Build history of the part. All positions in model axes, mm. Give positions to 0.01 mm unless a question says otherwise; leave off trailing zeros. Order: outer loops, then holes, each group sorted by start corner. A loop starts at its lowest first (then second) coordinate and runs counter-clockwise, first axis right, second up. Notation, with made-up numbers: M 37.25,-32 L 62.25,-32 A28 ccw 62.25,-5 Z; hole C 12.25,77.5 d9. An arc over 180 degrees is marked long. Answer as CSV lines item,"result".
from build123d import *

# Parameters (mm, degrees)
SKETCH1_R      = 1.1303
SKETCH1_R_2    = 1.130299999
EXTRUDE1_DEPTH = 12.7
SKETCH2_R      = 3.810000001
SKETCH2_R_2    = 1.130299999
EXTRUDE2_DEPTH = 17.145


with BuildPart() as part:
    # Sketch1 → Extrude1 (new body)
    with BuildSketch(Plane.XY):
        with BuildLine():
            Line((286.542223003, 20.061166103), (324.474632327, -15.639737839))
            ThreePointArc((324.474632327, -15.639737839), (329.813577235, -15.525304753), (329.793827414, -10.185170147))
            Line((329.793827414, -10.185170147), (297.063524693, 22.885170148))
            ThreePointArc((297.063524693, 22.885170148), (291.649695142, 22.043861139), (286.542223003, 20.061166103))
        make_face()
        with Locations((296.613066371, 17.154306926)):
            Circle(SKETCH1_R, mode=Mode.SUBTRACT)
        with Locations((327.08586457, -12.865289034)):
            Circle(SKETCH1_R_2, mode=Mode.SUBTRACT)
    extrude(amount=EXTRUDE1_DEPTH)

    # Sketch2 → Extrude2 (add)
    with BuildSketch(Plane.XY):
        with Locations(Location((327.08586457, -12.865289034, 0), (0, 0, 226.735854521))):
            Circle(SKETCH2_R)
        with Locations((327.08586457, -12.865289034)):
            Circle(SKETCH2_R_2, mode=Mode.SUBTRACT)
    extrude(amount=EXTRUDE2_DEPTH)


solid = part.part
Item 1: Probe line 1 along Z through (x, y) = (301, 9); line 2 along X through (y, z) = (-13.5, 7.5); line 3 along X through (y, z) = (-5, 1). List the from-to ranges inside material, lowest first. Write a range as from..to.
Geometry says:
line 1,"z = 0..12.7"
line 2,"x = 322.2..326.15, 328.02..330.84"
line 3,"x = 313.17..324.66"
Item 2: Band-saw the part on D-D (x = 307). Give the cut face in (y, z).
Geometry says:
outline,"M 0.81,0 L 12.85,0 L 12.85,12.7 L 0.81,12.7 Z"
Item 3: Pull direction Y, two halves, no side cores. Call faces 1 (the cylindrical face through (330.18, -15.09, 10.36)), 2 (the flat face through (310, 5, 0)), 3 (the cylindrical face through (328.13, -13.3, 8.45)): released by +Y, released by -Y, zero draft, split by the parting line, or undercut.
Geometry says:
face 1,"split by the parting line"
face 2,"zero draft"
face 3,"undercut"
Item 4: Band-saw the part on A-A (z = 2.5). Give the cut face in (x, y).
Geometry says:
outline,"M 286.54,20.06 L 324.47,-15.64 A3.81 ccw 329.79,-10.19 L 297.06,22.89 A25.4 ccw Z; hole C 296.61,17.15 d2.26; hole C 327.09,-12.87 d2.26"
Item 5: Band-saw the part on C-C (z = 14.25). Give the cut face in (x, y), and give its area (3 significant figures).
Geometry says:
outline,"C 327.09,-12.87 d7.62; hole C 327.09,-12.87 d2.26"
area,"41.6 mm2"
Item 6: Drop flat-ended pins along their axis: pin 1 (4 mm diameter, centred on x = 319, z = 2.5, fed in from +Y); pin 2 (2 mm diameter, centred on x = 312, z = 2, fed in from -Y); pin 3 (4 mm diameter, centred on x = 313, z = 11.5, fed in from +Y). Give the stop position or say it passes through.
Geometry says:
pin 1,"stops at y = 2.74"
pin 2,"stops at y = -4.84"
pin 3,"stops at y = 8.8"
Item 7: Band-saw the part on B-B (y = -13.5). Give the cut face in (x, z) (3 decimals), and give its area (3 significant figures).
Geometry says:
outline,"M 322.201,0 L 326.151,0 L 326.151,17.145 L 323.329,17.145 L 323.329,12.7 L 322.201,12.7 Z; M 328.021,0 L 330.843,0 L 330.843,17.145 L 328.021,17.145 Z"
area,"111 mm2"
